Part model, mm, in its own coordinate system. Give positions to 0.01 mm unless a question says otherwise; leave off trailing zeros. Write each loop counter-clockwise with the first axis right and the second up, starting at its lowest first coordinate (ties: lowest second). Pieces come first, ordered by that corner, then holes. Notation, with made-up numbers: (61.25, 56.25) - (103.25, 56.25) arc R16 ccw to (103.25, 66.25) - close; hole circle Ø6 at (-13, 64.5). An arc over 180 degrees is marked (long way). Answer in a Markdown table with one row per item. Add a question column.
1. Probe line 1 along Y through (x, z) = (0, 4); line 2 along X through (y, z) = (-70, 4.25); line 3 along Y through (x, z) = (8, 5.5). List the from-to ranges inside material, lowest first.
2. Band-saw the part on D-D on z = -5.75. State how many separate pieces and enclosed holes the cut face has, plus the area to 3 significant figures.
3. Band-saw the part on C-C on x = -235. Write the cut outline in (y, z), plus the area to 3 significant figures.
4. Band-saw the part on B-B on x = 0. Write the cut outline in (y, z).
5. Drop flat-ended pins along their axis: pin 1 Ø10 at (x, z) = (-163.5, -1) entering from +Y; pin 2 Ø10 at (x, z) = (114.5, 1) entering from +Y; pin 3 Ø4 at (x, z) = (-31, 3.5) entering from -Y. Give the stop position or say it passes through.
6. Band-saw the part on A-A on y = -70. Write the cut outline in (x, z), plus the area to 3 significant figures.
Autodesk Inventor part; units mm, degrees
ref_plane "YZ Plane" through (0, 0, 0) normal (1, 0, 0) x (0, 1, 0)
ref_plane "XZ Plane" through (0, 0, 0) normal (0, 1, 0) x (-1, 0, 0)
ref_plane "XY Plane" through (0, 0, 0) normal (0, 0, 1) x (1, 0, 0)
sketch "Sketch1" plane through (0, 0, 0) normal (0, 0, 1) x (1, 0, 0)
  circle A0 centre (0, 0) radius 20
  circle A1 centre (-235, -350) radius 11
  circle A2 centre (235, -350) radius 11
  arc A3 (257.6264, -370.5094) -> (260.9808, -323.1206) centre (233.6625, -345) ccw
  circle A4 centre (0.0008, -70) radius 11
  line L0 (70, -100) -> (-70, -100)
  line L1 (-80, -110) -> (-80, -290)
  line L2 (-70, -300) -> (70, -300)
  line L3 (80, -290) -> (80, -110)
  line L4 (80, -100) -> (-80, -300) construction
  line L5 (-80, -100) -> (80, -300) construction
  line L6 (0, 64.9697) -> (0, -492.5476)
  arc A5 (-260.9808, -323.1206) -> (-257.6264, -370.5094) centre (-233.6625, -345) ccw
  line L7 (-80, -110) -> (-70, -100)
  line L8 (80, -110) -> (70, -100)
  line L9 (70, -300) -> (80, -290)
  line L10 (-70, -300) -> (-80, -290)
  arc A6 (20, 40.3113) -> (-20, 40.3113) centre (0, 0) ccw
  circle A7 centre (0, -427.5724) radius 11
  line L11 (-257.6264, -370.5094) -> (-11, -457.5724)
  arc A8 (-11, -457.5724) -> (11, -457.5724) centre (0, -426.4123) ccw
  line L12 (257.6264, -370.5094) -> (11, -457.5724)
  line L13 (-11, -457.5724) -> (11, -457.5724) construction
  line L14 (268.5751, -347.4713) -> (268.5751, -36.5544)
  line L15 (246, -14.5226) -> (20, 40.3113)
  line L16 (-268.5751, -347.4713) -> (-268.5751, -36.5544)
  line L17 (-246, -14.5226) -> (-20, 40.3113)
  line L18 (-268.5751, -36.5544) -> (-268.5751, -20) construction
  line L19 (-268.5751, -20) -> (-246, -14.5226) construction
  spline S0 degree 2 poles (-268.5751, -36.5544) (-268.5751, -20) (-246, -14.5226) knots 1 1 1 2 2 2
  line L20 (268.5751, -36.5544) -> (268.5751, -20) construction
  line L21 (268.5751, -20) -> (246, -14.5226) construction
  spline S1 degree 2 poles (268.5751, -36.5544) (268.5751, -20) (246, -14.5226) knots 1 1 1 2 2 2
  point P0 (0, -200)
  point P1 (0, -200)
  dimension "d0" = 40
  dimension "d3" = 22
  dimension "d4" = 22
  dimension "d9" = 35
  dimension "d33" = 22
  dimension "d35" = 160
  dimension "d36" = 200
  dimension "d37" = 70
  dimension "d38" = 30
  dimension "d39" = 10
  dimension "d40" = 10
  dimension "d41" = 10
  dimension "d42" = 10
  dimension "d43" = 10
  dimension "d44" = 10
  dimension "d45" = 10
  dimension "d46" = 10
  dimension "d47" = 45
  dimension "d50" = 22
  dimension "d51" = 30
extrude "Extrusion3" add sketch "Sketch1" along normal mid plane 22.22 contours A0 L6 A6 L15 S1 L14 A3 L12 A8 A7 L2 L9 L3 L8 L0 A4 | A0 L6 A4 L0 L7 L1 L10 L2 A7 A8 L11 A5 L16 S0 L17 A6
equation "\"d40\" = d39"
equation "\"d42\" = d41"
equation "\"d43\" = d41"
equation "\"d44\" = d43"
equation "\"d45\" = d41"
equation "\"d46\" = d45"
properties part number "Corpo_Suporte_4_Cabos_Modelo2"
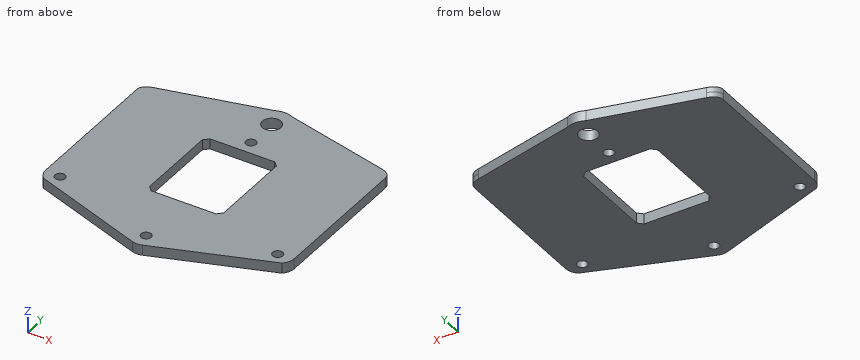
Values:
| question | item | result |
|---|---|---|
| 1 | line 1 | y = -459.46 to -438.57, -416.57 to -300, -100 to -81, -59 to -20, 20 to 45 |
| 1 | line 2 | x = -268.58 to -11, 11 to 268.58 |
| 1 | line 3 | y = -458.47 to -435.12, -420.02 to -300, -100 to -77.55, -62.45 to -18.33, 18.33 to 44.28 |
| 2 | separate pieces | 1 |
| 2 | enclosed holes | 6 |
| 2 | area | 194,000 mm² |
| 3 | outline | (-378.5, -11.11) - (-361, -11.11) - (-361, 11.11) - (-378.5, 11.11) - close; (-339, -11.11) - (-11.85, -11.11) - (-11.85, 11.11) - (-339, 11.11) - close |
| 3 | area | 7,660 mm² |
| 4 | outline | (-459.46, -11.11) - (-438.57, -11.11) - (-438.57, 11.11) - (-459.46, 11.11) - close; (-416.57, -11.11) - (-300, -11.11) - (-300, 11.11) - (-416.57, 11.11) - close; (-100, -11.11) - (-81, -11.11) - (-81, 11.11) - (-100, 11.11) - close; (-59, -11.11) - (-20, -11.11) - (-20, 11.11) - (-59, 11.11) - close; (20, -11.11) - (45, -11.11) - (45, 11.11) - (20, 11.11) - close |
| 5 | pin 1 | stops at y = 6.71 |
| 5 | pin 2 | stops at y = 18.6 |
| 5 | pin 3 | stops at y = -451.22 |
| 6 | outline | (-268.58, -11.11) - (-11, -11.11) - (-11, 11.11) - (-268.58, 11.11) - close; (11, -11.11) - (268.58, -11.11) - (268.58, 11.11) - (11, 11.11) - close |
| 6 | area | 11,400 mm² |
